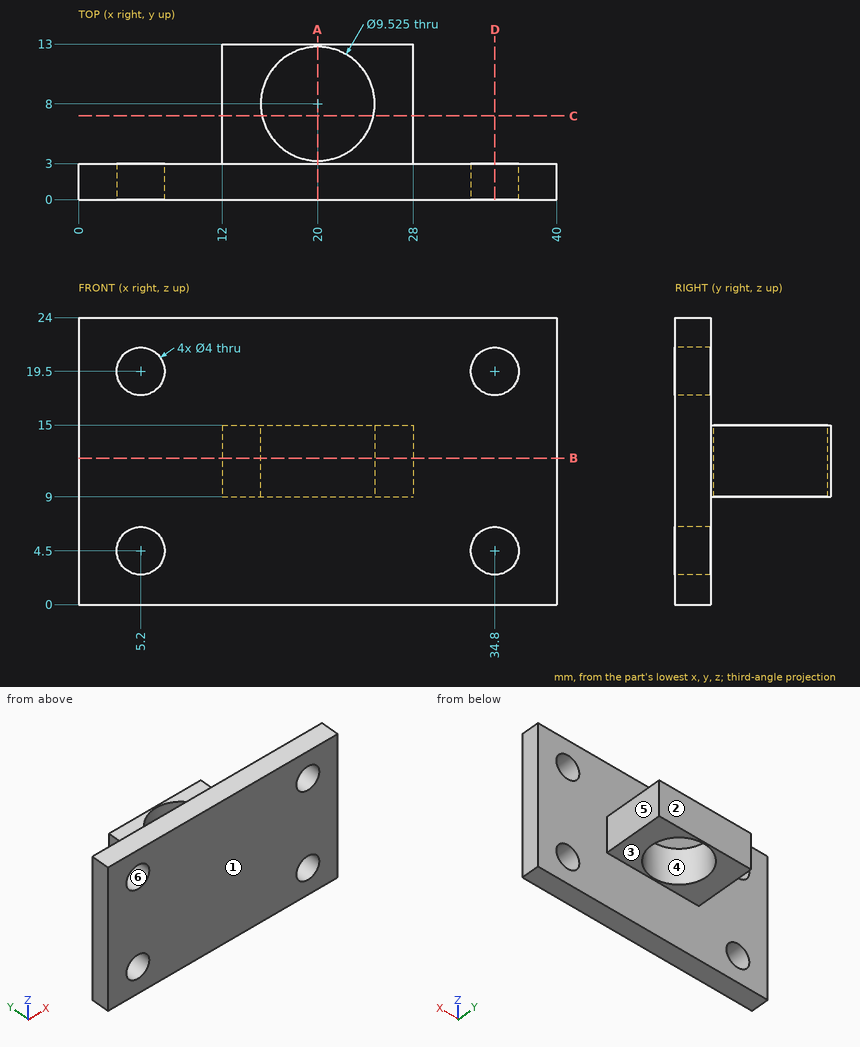
Could you check a few things on this drawing? It's one solid part, dimensions in mm from its lowest x, y, z. A direction names the side the tool comes from. Coordinates: 2 decimals unless noted, no trailing zeros. Write each loop counter-clockwise with the first axis right and the second up, starting at its lowest first coordinate (ties: lowest second). Pieces come first, ordered by that corner, then holes. Notation, with made-up numbers: M -2,-1.75 L 16,-1.75 A15 ccw 16,16.25 Z; hole C 11,-32.5 d9. An arc over 180 degrees is marked long. Answer as CSV lines item,"result". Start each with the question number.
Q1. If we mould it in two halves opening along Y, with no side actions, what happens to the marked faces 1, 2, 3 and 4? For each: pulls with the +Y half, pulls with the -Y half, needs draft (parallel to the pull), parting line crosses it, or undercut.
Q2. Suppose I cut it at A-A, the plane x = 20. List the corners of the cut face in (y, z) for me.
Q3. Suppose I cut it at B-B, the plane z = 12.25. List the corners of the cut face in (x, y) for me (1 decimal).
Q4. For the marked faces 5 and 6, which set-ups out of +Z, -Z, +X, -X, +Y, -Y let a thin tool reach every point of the face, with its end or its side?
Q5. Suppose I cut it at D-D, the plane x = 34.8. List the corners of the cut face in (y, z) for me, then the cut area to 3 significant figures.
Q6. Suppose I cut it at C-C, the plane y = 7. List the corners of the cut face in (x, z) for me, then the cut area to 3 significant figures.
Q7. I need wall thicknesses on probe 1 along Z at (x, y) = (34.8, 0.95); probe 2 along X at (y, z) = (1.4, 4.5); probe 3 along Y at (x, z) = (20, 11.8). Which ranges of each line are inside material? Lowest first, please. Write a range as [from, to].
Q8. Will these pins go through, and if not, where does the flat tip stop? pin 1 Ø5.5 at (x, y) = (20, 8) entering from +Z; pin 2 Ø6.5 at (x, z) = (5.2, 19.5) entering from -Y; pin 3 Ø2 at (y, z) = (8.5, 10) entering from -X; pin 4 Ø3 at (y, z) = (10.5, 11) entering from +X.
Entries:
1,face 1,"pulls with the -Y half"
1,face 2,"pulls with the +Y half"
1,face 3,"needs draft"
1,face 4,"undercut"
2,outline,"M 0,0 L 3,0 L 3,9 L 3.24,9 L 3.24,15 L 3,15 L 3,24 L 0,24 Z; M 12.76,9 L 13,9 L 13,15 L 12.76,15 Z"
3,outline,"M 0,0 L 40,0 L 40,3 L 28,3 L 28,13 L 12,13 L 12,3 L 0,3 Z; hole C 20,8 d9.5"
4,face 5,"+Z, -Z, +X, +Y"
4,face 6,"+Y, -Y"
5,outline,"M 0,0 L 3,0 L 3,2.5 L 0,2.5 Z; M 0,6.5 L 3,6.5 L 3,17.5 L 0,17.5 Z; M 0,21.5 L 3,21.5 L 3,24 L 0,24 Z"
5,area,"48.0 mm²"
6,outline,"M 12,9 L 15.34,9 L 15.34,15 L 12,15 Z; M 24.66,9 L 28,9 L 28,15 L 24.66,15 Z"
6,area,"40.1 mm²"
7,probe 1,"z = [0, 2.5], [6.5, 17.5], [21.5, 24]"
7,probe 2,"x = [0, 3.2], [7.2, 32.8], [36.8, 40]"
7,probe 3,"y = [0, 3.24], [12.76, 13]"
8,pin 1,"passes through"
8,pin 2,"stops at y = 0"
8,pin 3,"stops at x = 12"
8,pin 4,"stops at x = 28"
